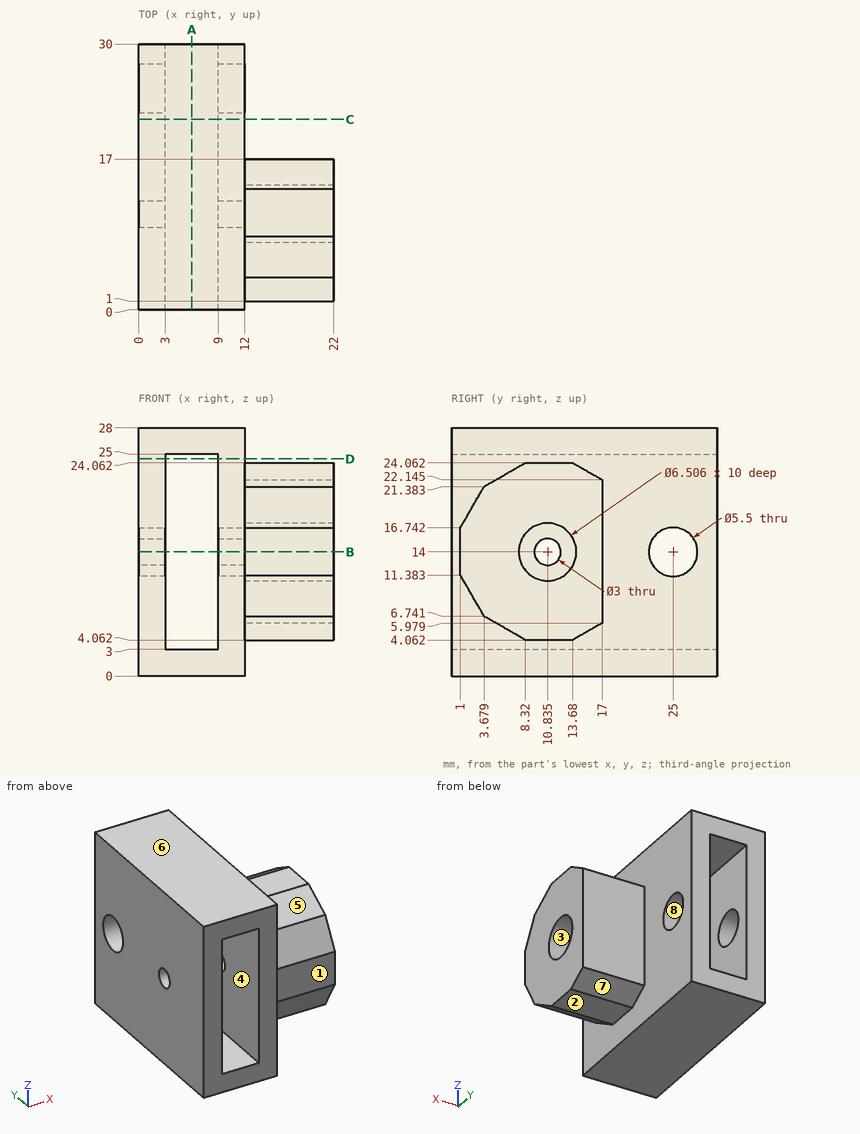
The figure shows three views and two pictorial views of one solid part (mm, origin at its lowest corner). Answer the questions. A direction names the side the tool comes from. Round coordinates to 2 decimals unless told otherwise and drop trailing zeros. Write each loop counter-clockwise with the first axis right and the second up, starting at its lowest first coordinate (ties: lowest second). Pieces come first, ordered by that corner, then holes. Notation, with made-up numbers: (-3.5, 75.25) - (3.5, 75.25) arc R29 cw to (3.5, 107.25) - close; hole circle Ø7 at (85.5, -18). An arc over 180 degrees is marked (long way). One line per question, with ' | ' between items. Start each with the question number.
1. Section D-D (z = 24.5) is taken. Determine the outline of the cut face in (x, y), and give its area (3 significant figures).
2. For the marked faces 1, 2, 3, 4 and 5, determine the directions among +Z, -Z, +X, -X, +Y, -Y from which every point of the face is accessible in a straight line to the end or side of a thin tool.
3. Each of these flat-tipped pins is pushed along its axis until it touches: pin 1 (2 mm diameter, centred on x = 8.5, z = 7, fed in from -Y); pin 2 (9 mm diameter, centred on y = 25, z = 14, fed in from +X); pin 3 (2.5 mm diameter, centred on x = 19.5, y = 10.5, fed in from -Z); pin 4 (4 mm diameter, centred on x = 18, z = 10.5, fed in from +Y). Where does it stop, or does it pass through?
4. Section C-C (y = 21.5) is taken. Determine the outline of the cut face in (x, z).
5. Section B-B (z = 14) is taken. Give the number of separate pieces and of enclosed holes in the cut face, and give its area (3 significant figures).
6. Section A-A (x = 6) is taken. Determine the outline of the cut face in (y, z).
7. For a pull along Y with two mould halves and no side action, classify the marked faces 6, 7 and 8 as +Y half, -Y half, draft (parallel to the pull), parting line (faces both ways), or undercut.
8. Find the intervals of material crossed by probe 1 along Z at (x, y) = (6.25, 22.25); probe 2 along X at (y, z) = (21.5, 9.75); probe 3 along Y at (x, z) = (16.5, 14), in increasing order. Write a range as [from, to].
Filled in:
1) outline: (0, 0) - (3, 0) - (3, 30) - (0, 30) - close; (9, 0) - (12, 0) - (12, 30) - (9, 30) - close | area: 180 mm²
2) face 1: +Z, -Z, +X, -Y | face 2: -Z, +X, +Y, -Y | face 3: +X | face 4: +Y, -Y | face 5: +Z, +X, -Y
3) pin 1: y = 0 | pin 2: x = 12 | pin 3: z = 4.06 | pin 4: y = 17
4) outline: (0, 0) - (12, 0) - (12, 28) - (0, 28) - close; hole (3, 3) - (9, 3) - (9, 25) - (3, 25) - close
5) separate pieces: 6 | enclosed holes: 0 | area: 224 mm²
6) outline: (0, 0) - (30, 0) - (30, 3) - (0, 3) - close; (0, 25) - (30, 25) - (30, 28) - (0, 28) - close
7) face 6: draft | face 7: +Y half | face 8: undercut
8) probe 1: [0, 3], [25, 28] | probe 2: [0, 3], [9, 12] | probe 3: [1, 7.58], [14.09, 17]
